Input: part model. Units: mm. Frame: model coordinates. A direction names the side the tool comes from. Round coordinates to 2 decimals unless told otherwise and drop trailing zeros. Write each loop counter-clockwise with the first axis right and the second up, starting at its lowest first coordinate (ties: lowest second). Pieces come first, ordered by that corner, then holes. Notation, with made-up numbers: (46.5, -20) -> (64.5, -20) arc R20 ccw to (64.5, -13) -> close; hole circle Ø6 at (22, -0.75). An arc over 180 degrees is marked (long way). Use CSV: the item, a comma, the result in double quotes.
```python
from build123d import *

# Parameters (mm, degrees)
F0_W     = 18.995181
F0_H     = 18.995181
F1_DEPTH = 37.9984
F0_W_2   = 18.995179
F2_DEPTH = 18.9992


with BuildPart() as f1:
    # F0 (on Front) → F1 (new body)
    with BuildSketch(Plane.XZ):
        with Locations((-9.49759, 9.49759)):
            Rectangle(F0_W, F0_H)
        with Locations((-9.49759, -9.49759)):
            Rectangle(F0_W, F0_H)
    extrude(amount=-F1_DEPTH)

    # F0 (on Front) → F2 (join)
    with BuildSketch(Plane.XZ):
        with Locations((9.49759, 9.49759)):
            Rectangle(F0_W_2, F0_H)
    extrude(amount=-F2_DEPTH)


solid = f1.part
```
Item 1: Line query: line 1 (Z direction, x = 14, y = 17); line 2 (X direction, y = 23.5, z = -16.5). Output: solid intervals per line, ascending.
Worked answers:
line 1,"z = 0 to 19"
line 2,"x = -19 to 0"
Item 2: Section query B-B on z = 11.5. Return the cut outline in (x, y), plus the area to 3 significant figures.
Worked answers:
outline,"(-19, 0) -> (19, 0) -> (19, 19) -> (0, 19) -> (0, 38) -> (-19, 38) -> close"
area,"1,080 mm²"
Item 3: Section query D-D on y = 23.5. Return the cut outline in (x, z), plus the area to 3 significant figures.
Worked answers:
outline,"(-19, -19) -> (0, -19) -> (0, 19) -> (-19, 19) -> close"
area,"722 mm²"
Item 4: First-contact query: pin 1 Ø8 at (y, z) = (9.5, -13.5) entering from +X; pin 2 Ø21 at (x, y) = (13, 9) entering from -Z; pin 3 Ø9.5 at (x, z) = (6, 12) entering from +Y. Flat tips, straight axial feed; report the tip coordinate or a pass-through.
Worked answers:
pin 1,"stops at x = 0"
pin 2,"stops at z = 0"
pin 3,"stops at y = 19"
Item 5: Set-up query: faces 1 (the face through (9, 9, 0)), 2 (the face through (-4, 15, 18.995)), 3 (the face through (9, 18.999, 10)). Return all of +Z, -Z, +X, -X, +Y, -Y with unobstructed straight access to the full face (end or side cutting, diameter ignored); none if empty.
Worked answers:
face 1,"-Z, +X, +Y, -Y"
face 2,"+Z, +X, -X, +Y, -Y"
face 3,"+Z, -Z, +X, +Y"
Item 6: Section query C-C on x = 10. Return the cut outline in (y, z).
Worked answers:
outline,"(0, 0) -> (19, 0) -> (19, 19) -> (0, 19) -> close"
Item 7: Section query A-A on y = 16. Return the cut outline in (x, z).
Worked answers:
outline,"(-19, -19) -> (0, -19) -> (0, 0) -> (19, 0) -> (19, 19) -> (-19, 19) -> close"
